Here's how the part is built. I have some questions about the finished solid (model axes, mm). Face numbers are marked on the shaded views. Round coordinates to 2 decimals unless told otherwise and drop trailing zeros. Write each loop counter-clockwise with the first axis right and the second up, starting at its lowest first coordinate (ties: lowest second). Pieces come first, ordered by that corner, then holes. Notation, with made-up numbers: (-34, -7.5) - (-22, -7.5) arc R9 ccw to (-22, 4.5) - close; hole circle Ø4 at (-32, -8). An arc over 180 degrees is marked (long way). One line per item, written item: value. Start each with the question number.
Item 1: If I drill on line 1 (Z direction, x = -26.1, y = 0); line 2 (Y direction, x = 0, z = 1.05); line 3 (Z direction, x = 0.5, y = 23.5), over which ranges is the centre line in solid material (lowest first)?
Item 2: Imagine slicing it at D-D, the plane x = -9. Please give me the cut outline in (y, z).
Item 3: For P1, Ø5, axis at x = 12.5, z = 3.5, coming from the +Y side; P2, Ø2, axis at x = -18.5, z = 5, coming from the +Y side; P3, Ø1.5, axis at y = 7.5, z = 8, coming from the -X side, each with a flat end and sliding along its axis, tell me the tip position at first contact or that it passes through.
Item 4: Imagine slicing it at C-C, the plane z = 5.5. Please give me the cut outline in (x, y), then the cut area to 3 significant figures.
Item 5: Imagine slicing it at A-A, the plane y = 0. Please give me the cut outline in (x, z).
Item 6: Thinking about a two-plate mould opening in Z: for the marked faces 1, 2 and 3, which applies, released by +Z, released by -Z, zero draft, split by the parting line, or undercut?
```python
from build123d import *

# Parameters (mm, degrees)
SKETCH1_R           = 28.5
SKETCH1_R_2         = 21.5
EXTRUDE_THIN1_DEPTH = 11
CUT_EXTRUDE1_START  = -1.95
SKETCH2_R           = 23.55
CUT_EXTRUDE1_DEPTH  = 7.1
SKETCH3_R           = 1.5
CUT_EXTRUDE2_DEPTH  = 42.779181419
CIRPATTERN1_COUNT   = 2
CIRPATTERN1_ANGLE   = 90


with BuildPart() as part:
    # Sketch1 → Extrude-Thin1 (new body)
    with BuildSketch(Plane(origin=(0, 0, 0), x_dir=(0, 1, 0), z_dir=(0, 0, 1))):
        Circle(SKETCH1_R)
        Circle(SKETCH1_R_2, mode=Mode.SUBTRACT)
    extrude(amount=EXTRUDE_THIN1_DEPTH)

    # Sketch2 → Cut-Extrude1 (cut)
    with BuildSketch(Plane(origin=(0, 0, 0), x_dir=(1, 0, 0), z_dir=(0, 0, -1)).offset(CUT_EXTRUDE1_START)):
        with Locations(Location((0, 0, 0), (0, 0, 180))):
            Circle(SKETCH2_R)
    extrude(amount=-CUT_EXTRUDE1_DEPTH, mode=Mode.SUBTRACT)

    # Sketch3 → Cut-Extrude2 (cut, symmetric)
    with BuildSketch(Plane.YZ):
        with Locations(Location((0, 5.5, 0), (0, 0, 270))):
            Circle(SKETCH3_R)
    cut_extrude2 = extrude(amount=CUT_EXTRUDE2_DEPTH, both=True, mode=Mode.SUBTRACT)

    # CirPattern1: Cut-Extrude2 ×2 about axis
    cirpattern1_axis = Axis((0, 0, 9.05), (0, 0, -1))
    for i in range(1, CIRPATTERN1_COUNT):
        add(cut_extrude2.rotate(cirpattern1_axis, i * CIRPATTERN1_ANGLE / (CIRPATTERN1_COUNT - 1)), mode=Mode.SUBTRACT)


solid = part.part
```
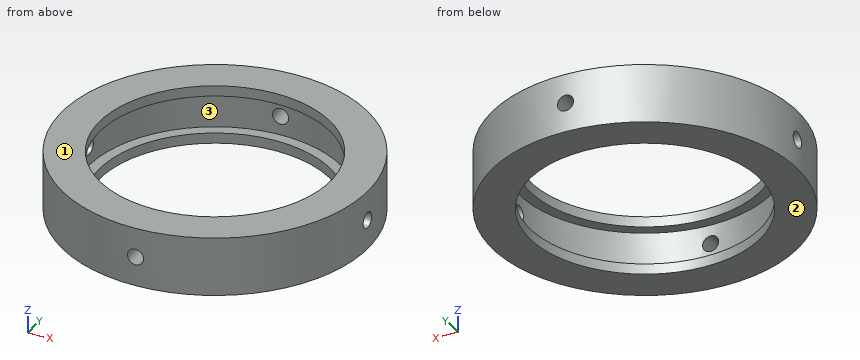
Values follow:
1. line 1: z = 0 to 4, 7 to 11
1. line 2: y = -28.5 to -21.5, 21.5 to 28.5
1. line 3: z = 0 to 1.95, 9.05 to 11
2. outline: (-27.04, 0) - (-19.53, 0) - (-19.53, 1.95) - (-21.76, 1.95) - (-21.76, 9.05) - (-19.53, 9.05) - (-19.53, 11) - (-27.04, 11) - close; (19.53, 0) - (27.04, 0) - (27.04, 11) - (19.53, 11) - (19.53, 9.05) - (21.76, 9.05) - (21.76, 1.95) - (19.53, 1.95) - close
3. P1: stops at y = 26.69
3. P2: stops at y = 22.49
3. P3: stops at x = -27.69
4. outline: (-28.46, -1.5) arc R28.5 ccw to (-1.5, -28.46) - (-1.5, -23.5) arc R23.55 cw to (-23.5, -1.5) - close; (-28.46, 1.5) - (-23.5, 1.5) arc R23.55 cw to (-1.5, 23.5) - (-1.5, 28.46) arc R28.5 ccw to start; (1.5, -28.46) arc R28.5 ccw to (28.46, -1.5) - (23.5, -1.5) arc R23.55 cw to (1.5, -23.5) - close; (1.5, 23.5) arc R23.55 cw to (23.5, 1.5) - (28.46, 1.5) arc R28.5 ccw to (1.5, 28.46) - close
4. area: 750 mm^2
5. outline: (-28.5, 0) - (-21.5, 0) - (-21.5, 1.95) - (-23.55, 1.95) - (-23.55, 4) - (-28.5, 4) - close; (-28.5, 7) - (-23.55, 7) - (-23.55, 9.05) - (-21.5, 9.05) - (-21.5, 11) - (-28.5, 11) - close; (21.5, 0) - (28.5, 0) - (28.5, 4) - (23.55, 4) - (23.55, 1.95) - (21.5, 1.95) - close; (21.5, 9.05) - (23.55, 9.05) - (23.55, 7) - (28.5, 7) - (28.5, 11) - (21.5, 11) - close
6. face 1: released by +Z
6. face 2: released by -Z
6. face 3: undercut
